For this review, take the finished solid that the model builds, in its own axes (mm). A direction names the side the tool comes from. Coordinates: 2 decimals unless noted, no trailing zeros. Loops run counter-clockwise (first coordinate to the right, second up) from the corner with the lowest first, then second, coordinate; pieces in that order, holes last. Notation, with made-up numbers: (-40, -12.75) -> (18, -12.75) arc R22 ccw to (18, 14.25) -> close; hole circle Ø10 at (15, 4.5). An arc over 180 degrees is marked (long way). Answer in a Markdown table with one row per item.
from build123d import *

# Parameters (mm, degrees)
BOSS_EXTRUDE1_DEPTH = 80
SKETCH2_W           = 68
SKETCH2_H           = 12
CUT_EXTRUDE1_DEPTH  = 60
FILLET1_R           = 10
CUT_EXTRUDE6_DEPTH  = 60
SKETCH6_R           = 29.25
CUT_EXTRUDE7_DEPTH  = 95
SKETCH7_R           = 3
CUT_EXTRUDE8_DEPTH  = 41
CUT_EXTRUDE9_START  = -20
CUT_EXTRUDE9_DEPTH  = 4
CUT_EXTRUDE10_DEPTH = 30
CUT_EXTRUDE11_START = -90
CUT_EXTRUDE11_DEPTH = 90
SKETCH11_R          = 4.15
CUT_EXTRUDE12_DEPTH = 18
SKETCH12_R          = 4.15
CUT_EXTRUDE13_DEPTH = 18


with BuildPart() as part:
    # Sketch1 → Boss-Extrude1 (new body)
    with BuildSketch(Plane.XY):
        Polygon((25, 0), (-25, 0), (-34, -50), (-34, -160), (34, -160), (34, -50), align=None)
    extrude(amount=BOSS_EXTRUDE1_DEPTH)

    # Sketch2 → Cut-Extrude1 (cut)
    with BuildSketch(Plane.XZ.offset(160)):
        with Locations((0, 74)):
            Rectangle(SKETCH2_W, SKETCH2_H)
    extrude(amount=-CUT_EXTRUDE1_DEPTH, mode=Mode.SUBTRACT)

    # Fillet1
    fillet1_edges = [part.edges().sort_by_distance(p)[0] for p in [
        (0, -100, 68),
    ]]
    fillet(fillet1_edges, radius=FILLET1_R)

    # Sketch5 → Cut-Extrude6 (cut)
    with BuildSketch(Plane.XY.offset(80)):
        with BuildLine():
            Line((17.1, -45.5), (6.9, -45.5))
            ThreePointArc((6.9, -45.5), (5.061522369, -44.738477631), (4.3, -42.9))
            Line((4.3, -42.9), (4.3, -41.72))
            ThreePointArc((4.3, -41.72), (5.120101013, -39.740101013), (7.1, -38.92))
            Line((7.1, -38.92), (7.460539391, -38.92))
            ThreePointArc((7.460539391, -38.92), (9.09596662, -37.871916072), (8.826877189, -35.948197533))
            Line((8.826877189, -35.948197533), (5.457008123, -32.578328466))
            ThreePointArc((5.457008123, -32.578328466), (4.988893203, -32.349986186), (4.479421839, -32.458202195))
            ThreePointArc((4.479421839, -32.458202195), (0, -33.7), (-4.479421839, -32.458202195))
            ThreePointArc((-4.479421839, -32.458202195), (-4.988893203, -32.349986186), (-5.457008123, -32.578328466))
            Line((-5.457008123, -32.578328466), (-8.826877189, -35.948197533))
            ThreePointArc((-8.826877189, -35.948197533), (-9.09596662, -37.871916072), (-7.460539391, -38.92))
            Line((-7.460539391, -38.92), (-7.1, -38.92))
            ThreePointArc((-7.1, -38.92), (-5.120101013, -39.740101013), (-4.3, -41.72))
            Line((-4.3, -41.72), (-4.3, -42.9))
            ThreePointArc((-4.3, -42.9), (-5.061522369, -44.738477631), (-6.9, -45.5))
            Line((-6.9, -45.5), (-17.1, -45.5))
            ThreePointArc((-17.1, -45.5), (-19.504163056, -44.504163056), (-20.5, -42.1))
            Line((-20.5, -42.1), (-20.5, -32.118179099))
            ThreePointArc((-20.5, -32.118179099), (-19.895099696, -30.212814465), (-18.116592311, -29.3))
            Line((-18.116592311, -29.3), (-16.72, -29.3))
            ThreePointArc((-16.72, -29.3), (-14.740101013, -30.120101013), (-13.92, -32.1))
            Line((-13.92, -32.1), (-13.92, -32.460539391))
            ThreePointArc((-13.92, -32.460539391), (-12.871916072, -34.09596662), (-10.948197533, -33.826877189))
            Line((-10.948197533, -33.826877189), (-7.578328467, -30.457008123))
            ThreePointArc((-7.578328467, -30.457008123), (-7.349986186, -29.988893203), (-7.458202195, -29.479421839))
            ThreePointArc((-7.458202195, -29.479421839), (-8.7, -25), (-7.458202195, -20.520578161))
            ThreePointArc((-7.458202195, -20.520578161), (-7.349986186, -20.011106797), (-7.578328467, -19.542991877))
            Line((-7.578328467, -19.542991877), (-10.948197533, -16.173122811))
            ThreePointArc((-10.948197533, -16.173122811), (-12.871916072, -15.90403338), (-13.92, -17.539460609))
            Line((-13.92, -17.539460609), (-13.92, -17.9))
            ThreePointArc((-13.92, -17.9), (-14.740101013, -19.879898987), (-16.72, -20.7))
            Line((-16.72, -20.7), (-18.116592311, -20.7))
            ThreePointArc((-18.116592311, -20.7), (-19.895099696, -19.787185535), (-20.5, -17.881820901))
            Line((-20.5, -17.881820901), (-20.5, -7.9))
            ThreePointArc((-20.5, -7.9), (-19.504163056, -5.495836944), (-17.1, -4.5))
            Line((-17.1, -4.5), (-7.1, -4.5))
            Line((-7.1, -4.5), (7.1, -4.5))
            Line((7.1, -4.5), (17.1, -4.5))
            ThreePointArc((17.1, -4.5), (19.504163056, -5.495836944), (20.5, -7.9))
            Line((20.5, -7.9), (20.5, -18.1))
            Line((20.5, -18.1), (20.5, -31.9))
            Line((20.5, -31.9), (20.5, -42.1))
            ThreePointArc((20.5, -42.1), (19.504163056, -44.504163056), (17.1, -45.5))
        make_face()
    extrude(amount=-CUT_EXTRUDE6_DEPTH, mode=Mode.SUBTRACT)

    # Sketch6 → Cut-Extrude7 (cut)
    with BuildSketch(Plane.XZ.offset(160)):
        with Locations(Location((0, 34, 0), (0, 0, 270))):
            Circle(SKETCH6_R)
    extrude(amount=-CUT_EXTRUDE7_DEPTH, mode=Mode.SUBTRACT)

    # Sketch7 → Cut-Extrude8 (cut)
    with BuildSketch(Plane.XZ.offset(160)):
        with Locations(Location((-23.511300474, 57.511300474, 0), (0, 0, 270))):
            Circle(SKETCH7_R)
        with Locations(Location((23.511300474, 57.511300474, 0), (0, 0, 270))):
            Circle(SKETCH7_R)
        with Locations(Location((23.511300474, 10.488699526, 0), (0, 0, 270))):
            Circle(SKETCH7_R)
        with Locations(Location((-23.511300474, 10.488699526, 0), (0, 0, 270))):
            Circle(SKETCH7_R)
    extrude(amount=-CUT_EXTRUDE8_DEPTH, mode=Mode.SUBTRACT)

    # Sketch8 → Cut-Extrude9 (cut)
    with BuildSketch(Plane.XZ.offset(160).offset(CUT_EXTRUDE9_START)):
        Polygon((-26.450688166, 54.571912783), (-22.435409908, 53.496022217), (-19.496022217, 56.435409908), (-20.571912783, 60.450688166), (-20.571912783, 68), (-34, 68), (-34, 54.571912783), align=None)
        Polygon((20.571912783, 60.450688166), (19.496022217, 56.435409908), (22.435409908, 53.496022217), (26.450688166, 54.571912783), (34, 54.571912783), (34, 68), (20.571912783, 68), align=None)
        Polygon((26.450688166, 13.428087217), (22.435409908, 14.503977783), (19.496022217, 11.564590092), (20.571912783, 7.549311834), (20.571912783, 0), (34, 0), (34, 13.428087217), align=None)
        Polygon((-20.571912783, 7.549311834), (-19.496022217, 11.564590092), (-22.435409908, 14.503977783), (-26.450688166, 13.428087217), (-34, 13.428087217), (-34, 0), (-20.571912783, 0), align=None)
    extrude(amount=-CUT_EXTRUDE9_DEPTH, mode=Mode.SUBTRACT)

    # Sketch9 → Cut-Extrude10 (cut)
    with BuildSketch(Plane.XY.offset(80)):
        Polygon((4.185789452, -63.75), (-4.185789452, -63.75), (-8.371578903, -71), (-4.185789452, -78.25), (4.185789452, -78.25), (8.371578903, -71), align=None)
    extrude(amount=-CUT_EXTRUDE10_DEPTH, mode=Mode.SUBTRACT)

    # Sketch10 → Cut-Extrude11 (cut)
    with BuildSketch(Plane(origin=(0, -78.25, 0), x_dir=(1, 0, 0), z_dir=(0, 1, 0)).offset(CUT_EXTRUDE11_START)):
        with BuildLine():
            Line((-4.185789452, -62.948949319), (-4.185789452, -80))
            Line((-4.185789452, -80), (4.185789452, -80))
            Line((4.185789452, -80), (4.185789452, -62.948949319))
            ThreePointArc((4.185789452, -62.948949319), (0, -63.25), (-4.185789452, -62.948949319))
        make_face()
    extrude(amount=CUT_EXTRUDE11_DEPTH, mode=Mode.SUBTRACT)

    # Sketch11 → Cut-Extrude12 (cut)
    with BuildSketch(Plane(origin=(0, 0, 0), x_dir=(1, 0, 0), z_dir=(0, 1, 0))):
        with Locations(Location((0, -50, 0), (0, 0, 180))):
            Circle(SKETCH11_R)
    extrude(amount=-CUT_EXTRUDE12_DEPTH, mode=Mode.SUBTRACT)

    # Sketch12 → Cut-Extrude13 (cut)
    with BuildSketch(Plane.ZY.offset(-20.5)):
        with Locations((50, -25)):
            Circle(SKETCH12_R)
    extrude(amount=-CUT_EXTRUDE13_DEPTH, mode=Mode.SUBTRACT)


solid = part.part
Item 1: Take a section at A-A, the plane y = -25. State the section outline as (x, z) points, and give its area (3 significant figures).
Worked answers:
| item | result |
|---|---|
| outline | (-29.5, 0) -> (29.5, 0) -> (29.5, 45.85) -> (20.5, 45.85) -> (20.5, 20) -> (-8.7, 20) -> (-8.7, 80) -> (-29.5, 80) -> close; (20.5, 54.15) -> (29.5, 54.15) -> (29.5, 80) -> (20.5, 80) -> close |
| area | 2,890 mm² |
Item 2: The part is to be moulded in two halves that separate along Z. For faces 6 (the flat face through (29.563, -25.35, 39.44)), 7 (the flat face through (0, -65, 34)), 8 (the cylindrical face through (-18.88, -102.85, 71.01)), say which applies: +Z half, -Z half, draft (parallel to the pull), parting line (faces both ways), or undercut.
Worked answers:
| item | result |
|---|---|
| face 6 | draft |
| face 7 | undercut |
| face 8 | +Z half |
Item 3: Insertion check: pin 1 (5 mm diameter, centred on y = -37.5, z = 63.5, fed in from +X); pin 2 (1.2 mm diameter, centred on y = -137, z = 2.5, fed in from -X); pin 3 (5 mm diameter, centred on x = -23.51, z = 57.51, fed in from -Y). Each pin has a flat end and moves straight along its axis. Give the tip position at first contact, or say it passes through.
Worked answers:
| item | result |
|---|---|
| pin 1 | x = 32.2 |
| pin 2 | x = -20.57 |
| pin 3 | y = -119 |
Item 4: For L1, parallel to Y at x = -17.5, z = 25; L2, parallel to Y at x = 5.5, z = 50.5; L3, parallel to Y at x = 7.5, z = 70, list the stretches that pass through material, from the lowest coordinate up.
Worked answers:
| item | result |
|---|---|
| L1 | -65 to -45.48, -29.3 to -20.7, -4.52 to 0 |
| L2 | -65 to -45.09, -39.42 to -32.62, -4.5 to 0 |
| L3 | -104 to -72.51, -69.49 to -45.5, -38.92 to -34.62, -4.5 to 0 |
Item 5: For faces 1 (the cylindrical face through (-8.7, -25.1, 50.4)), 2 (the flat face through (20.026, -138.028, 9.585)), 3 (the flat face through (0, -63.75, 65)), 4 (the flat face through (-20.04, -138.03, 9.53)), 5 (the flat face through (24, -119, 58)), list the 3-axis set-ups (+Z, -Z, +X, -X, +Y, -Y) from which the entire face can be reached by the end or side of a thin tool; tool diameter is ignored.
Worked answers:
| item | result |
|---|---|
| face 1 | +Z |
| face 2 | +X |
| face 3 | +Z, -Y |
| face 4 | -X |
| face 5 | -Y |
Item 6: Take a section at B-B, the plane y = -112. State the section outline as (x, z) points.
Worked answers:
| item | result |
|---|---|
| outline | (-34, 0) -> (34, 0) -> (34, 68) -> (4.19, 68) -> (4.19, 62.95) arc R29.25 cw (long way) to (-4.19, 62.95) -> (-4.19, 68) -> (-34, 68) -> close |
